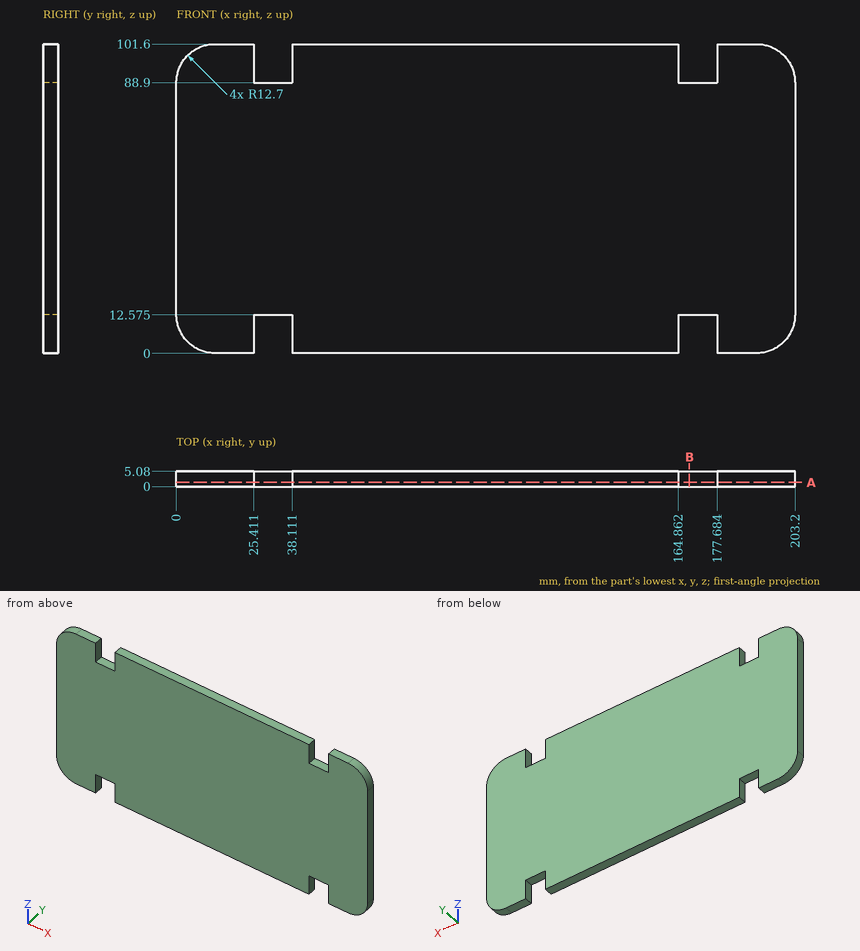
Check sheet for the drawn part. Datum: minimum x, y, z corner. Units: mm. Give positions to 0.01 mm unless a question says otherwise; leave off trailing zeros. Write each loop counter-clockwise with the first axis right and the second up, starting at its lowest first coordinate (ties: lowest second). Pieces come first, ordered by that corner, then holes. Notation, with made-up numbers: M 2.25,-29.5 L 55.25,-29.5 A30 cw 55.25,9.5 Z; hole C 16.25,-4.75 d1. An arc over 180 degrees is marked long. One line per question, with ' | ' between items.
1) Thickness scan on line 1 along X through (y, z) = (2.1, 91.5) (1 decimal); line 2 along X through (y, z) = (4.85, 94) (1 decimal); line 3 along Z through (x, y) = (174, 4.2) (1 decimal). Record the ranges inside material, lowest first. Write a range as [from, to].
Result:
line 1: x = [0.3, 25.4], [38.1, 164.9], [177.7, 202.9] | line 2: x = [1.1, 25.4], [38.1, 164.9], [177.7, 202.1] | line 3: z = [12.6, 88.9]
2) Section check B-B on x = 168.5. Enter the section's corners in (y, z) (1 decimal), plus the area to 3 significant figures.
Result:
outline: M 0,12.6 L 5.1,12.6 L 5.1,88.9 L 0,88.9 Z | area: 388 mm2
3) Section check A-A on y = 1.4. Enter the section's corners in (x, z) (1 decimal).
Result:
outline: M 0,12.7 A12.7 ccw 12.7,0 L 25.4,0 L 25.4,12.6 L 38.1,12.6 L 38.1,0 L 164.9,0 L 164.9,12.6 L 177.7,12.6 L 177.7,0 L 190.5,0 A12.7 ccw 203.2,12.7 L 203.2,88.9 A12.7 ccw 190.5,101.6 L 177.7,101.6 L 177.7,88.9 L 164.9,88.9 L 164.9,101.6 L 38.1,101.6 L 38.1,88.9 L 25.4,88.9 L 25.4,101.6 L 12.7,101.6 A12.7 ccw 0,88.9 Z
4) Gauge pin test, flat ends, axial feed: pin 1 Ø1.5 at (y, z) = (2, 6) entering from -X; pin 2 Ø1.5 at (y, z) = (2.5, 95) entering from -X; pin 3 Ø2.5 at (x, y) = (171.5, 2.5) entering from +Z. Record the tip position at first contact, or that the pin passes through.
Result:
pin 1: stops at x = 1.48 | pin 2: stops at x = 1.18 | pin 3: stops at z = 88.9
